For this review, take the finished solid that the model builds, in its own axes (mm). A direction names the side the tool comes from. Give positions to 0.01 mm unless a question says otherwise; leave off trailing zeros. Loops run counter-clockwise (first coordinate to the right, second up) from the corner with the lowest first, then second, coordinate; pieces in that order, holes last. Notation, with made-up numbers: (72, 40.25) - (111, 40.25) arc R21 cw to (111, 50.25) - close; hole circle Ø9 at (89.25, 88.5). An arc over 180 degrees is marked (long way). Answer in a Markdown table with one row per item.
```python
from build123d import *

# Parameters (mm, degrees)
SKETCH_1_W          = 30
SKETCH_1_H          = 25
EXTRUDE_1_DEPTH     = 10
FILLET_1_R          = 5
SKETCH_2_R          = 4
CUT_EXTRUDE_1_DEPTH = 14


with BuildPart() as part:
    # 草图1 → 凸台-拉伸1 (new body)
    with BuildSketch(Plane.XY):
        with BuildLine():
            ThreePointArc((-27.5, 0), (-31.353571801, 12.124355653), (-41.5, 19.798989873))
            ThreePointArc((-41.5, 19.798989873), (-44.948858447, 20.697569753), (-48.5, 21))
            ThreePointArc((-48.5, 21), (-63.349242405, 14.849242405), (-69.5, 0))
            ThreePointArc((-69.5, 0), (-63.349242405, -14.849242405), (-48.5, -21))
            ThreePointArc((-48.5, -21), (-44.948858447, -20.697569753), (-41.5, -19.798989873))
            ThreePointArc((-41.5, -19.798989873), (-31.353571801, -12.124355653), (-27.5, 0))
        make_face()
        with BuildLine():
            Line((39.5, 12.5), (-41.5, 19.798989873))
            ThreePointArc((-41.5, 19.798989873), (-31.353571801, 12.124355653), (-27.5, 0))
            ThreePointArc((-27.5, 0), (-31.353571801, -12.124355653), (-41.5, -19.798989873))
            Line((-41.5, -19.798989873), (39.5, -12.5))
            Line((39.5, -12.5), (39.5, 12.5))
        make_face()
        with Locations((54.5, 0)):
            Rectangle(SKETCH_1_W, SKETCH_1_H)
    extrude(amount=EXTRUDE_1_DEPTH)

    # 圆角1
    fillet_1_edges = [part.edges().sort_by_distance(p)[0] for p in [
        (69.5, 12.5, 5),
        (69.5, -12.5, 5),
    ]]
    fillet(fillet_1_edges, radius=FILLET_1_R)

    # 草图2 → 切除-拉伸1 (cut)
    with BuildSketch(Plane.XY.offset(10)):
        with Locations((-51.5, 0)):
            Circle(SKETCH_2_R)
    extrude(amount=-CUT_EXTRUDE_1_DEPTH, mode=Mode.SUBTRACT)


solid = part.part
```
1. We need section C-C, the plane y = -16.5. Give the boundary of the cut face in (x, z), and give its area (3 significant figures).
Values:
| item | result |
|---|---|
| outline | (-61.49, 0) - (-4.89, 0) - (-4.89, 10) - (-61.49, 10) - close |
| area | 566 mm^2 |
2. For faces 1 (the face through (52, -12.5, 5)), 2 (the face through (68.07, 11, 5.07)), list the 3-axis set-ups (+Z, -Z, +X, -X, +Y, -Y) from which the entire face can be reached by the end or side of a thin tool; tool diameter is ignored.
Values:
| item | result |
|---|---|
| face 1 | +Z, -Z, +X, -Y |
| face 2 | +Z, -Z, +X, +Y |
3. Clearance check with flat-ended pins moving along their axes: pin 1 (5 mm diameter, centred on y = -9.5, z = 4, fed in from -X); pin 2 (1.5 mm diameter, centred on y = -1, z = 6.5, fed in from -X); pin 3 (5 mm diameter, centred on x = -51.5, y = 0, fed in from +Z); pin 4 (1.5 mm diameter, centred on x = 55, z = 8, fed in from +Y). State where each tip first meets the part, or that it passes through.
Values:
| item | result |
|---|---|
| pin 1 | stops at x = -68.3 |
| pin 2 | stops at x = -69.5 |
| pin 3 | passes through |
| pin 4 | stops at y = 12.5 |
4. We need section B-B, the plane x = -51.5. Give the boundary of the cut face in (y, z), and give its area (3 significant figures).
Values:
| item | result |
|---|---|
| outline | (-20.78, 0) - (-4, 0) - (-4, 10) - (-20.78, 10) - close; (4, 0) - (20.78, 0) - (20.78, 10) - (4, 10) - close |
| area | 336 mm^2 |
5. We need section D-D, the plane x = 43. Give the boundary of the cut face in (y, z), and give its area (3 significant figures).
Values:
| item | result |
|---|---|
| outline | (-12.5, 0) - (12.5, 0) - (12.5, 10) - (-12.5, 10) - close |
| area | 250 mm^2 |
6. Wall thickness on line 1 (Y direction, x = 48.5, z = 1.75); line 2 (Y direction, x = -51.5, z = 2.5); line 3 (Y direction, x = 38.5, z = 3.25): over which ranges is each line inside the solid? List them lowest first. Write a range as [from, to].
Values:
| item | result |
|---|---|
| line 1 | y = [-12.5, 12.5] |
| line 2 | y = [-20.78, -4], [4, 20.78] |
| line 3 | y = [-12.59, 12.59] |
7. We need section A-A, the plane z = 3.5. Give the boundary of the cut face in (x, y), and give its area (3 significant figures).
Values:
| item | result |
|---|---|
| outline | (-41.5, -19.8) - (39.5, -12.5) - (64.5, -12.5) arc R5 ccw to (69.5, -7.5) - (69.5, 7.5) arc R5 ccw to (64.5, 12.5) - (39.5, 12.5) - (-41.5, 19.8) arc R21 ccw (long way) to start; hole circle Ø8 at (-51.5, 0) |
| area | 4,290 mm^2 |
8. Mouldability with a two-part tool opening along X and no side actions: class faces 3 (the face through (-47.685, 1.201, 5.07)), 4 (the face through (52, 12.5, 5)), 5 (the face through (-1.57, -16.2, 4.93)) as released by +X, released by -X, zero draft, split by the parting line, or undercut.
Values:
| item | result |
|---|---|
| face 3 | undercut |
| face 4 | zero draft |
| face 5 | released by +X |
